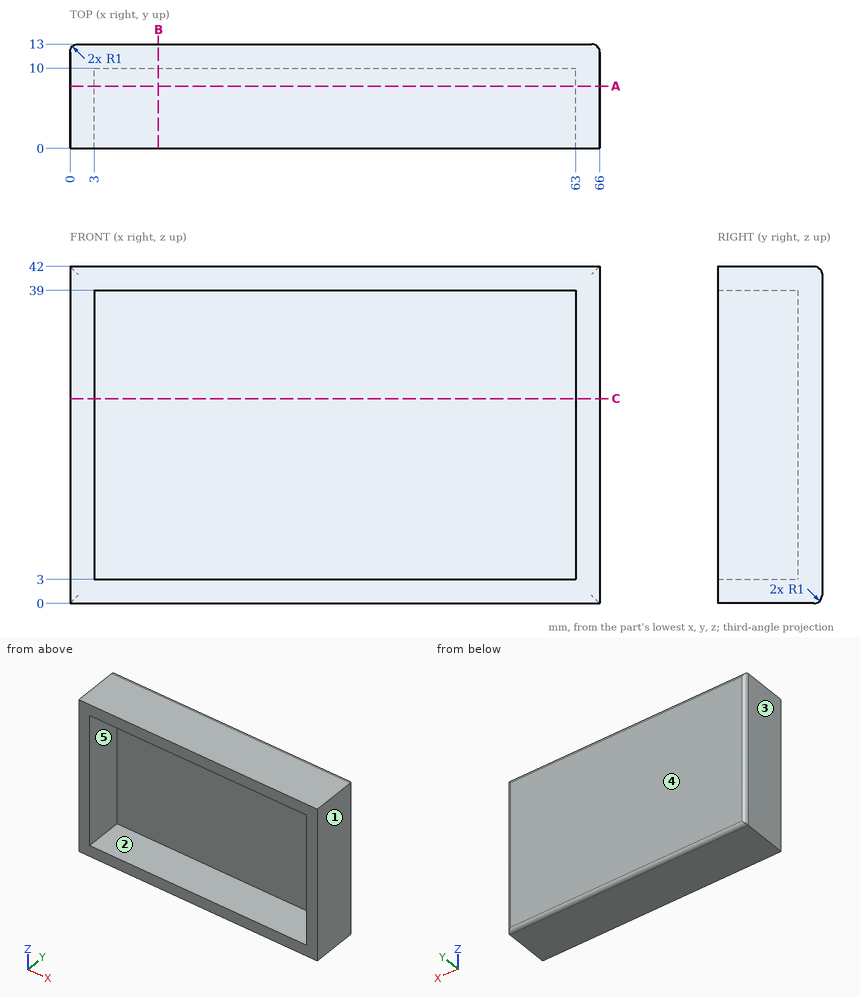
Study the drawing (mm; zero at the part's minimum x, y, z) and answer. A direction names the side the tool comes from. Round coordinates to 2 decimals unless told otherwise and drop trailing zeros. Order: outer loops, then holes, each group sorted by start corner. A loop starts at its lowest first (then second) coordinate and runs counter-clockwise, first axis right, second up. Notation, with made-up numbers: (-22.5, -32) - (-10.5, -32) arc R31 cw to (-10.5, 1) - close; hole circle Ø1 at (80, 76). An arc over 180 degrees is marked (long way). Use one line per item in the form item = value. Start each with the question number.
(1) For the marked faces 4 and 5, determine the directions among +Z, -Z, +X, -X, +Y, -Y from which every point of the face is accessible in a straight line to the end or side of a thin tool.
(2) The part is cut by section C-C (z = 25.5). Give the vertices of the cut face in (x, y).
(3) Find the intervals of material crossed by line 1 along X through (y, z) = (2, 25); line 2 along Z through (x, y) = (22, 3.5); line 3 along Y through (x, z) = (49.5, 21), in increasing order. Write a range as from..to.
(4) A flat-ended cylindrical pin translates along its axis: pin 1 Ø10 at (x, z) = (40.5, 26.5) entering from -Y. Find the tip coordinate at first contact, or state that the pin passes through.
(5) The part is cut by section B-B (x = 11). Give the vertices of the cut face in (y, z).
(6) Determine the mould class of the marked faces 1, 2 and 3 for opening direction X: +X half, -X half, draft (parallel to the pull), parting line (faces both ways), or undercut.
(7) The part is cut by section A-A (y = 7.75). Give the vertices of the cut face in (x, z), then the cut area to 3 significant figures.
Checked values:
q1.face_4 = +Z, -Z, +X, -X, +Y
q1.face_5 = -Y
q2.outline = (0, 0) - (3, 0) - (3, 10) - (63, 10) - (63, 0) - (66, 0) - (66, 12) arc R1 ccw to (65, 13) - (1, 13) arc R1 ccw to (0, 12) - close
q3.line_1 = 0..3, 63..66
q3.line_2 = 0..3, 39..42
q3.line_3 = 10..13
q4.pin_1 = 10
q5.outline = (0, 0) - (12, 0) arc R1 ccw to (13, 1) - (13, 41) arc R1 ccw to (12, 42) - (0, 42) - (0, 39) - (10, 39) - (10, 3) - (0, 3) - close
q6.face_1 = +X half
q6.face_2 = undercut
q6.face_3 = -X half
q7.outline = (0, 0) - (66, 0) - (66, 42) - (0, 42) - close; hole (3, 3) - (63, 3) - (63, 39) - (3, 39) - close
q7.area = 612 mm^2
